The listing builds one solid part. Answer for the finished solid, in the listing's coordinates (mm). A direction names the side the tool comes from. Round coordinates to 2 decimals unless told otherwise and drop trailing zeros. Order: outer loops, then holes, each group sorted by start corner. A loop starts at its lowest first (then second) coordinate and runs counter-clockwise, first axis right, second up. Notation, with made-up numbers: M 83,36.5 L 127,36.5 A16 cw 127,56.5 Z; hole C -37.5,20 d4. An arc over 180 degrees is marked long. Put each result on its own line as item: value. Start each with the question number.
1. The part is cut by section D-D (x = 110). Give the vertices of the cut face in (y, z), then the cut area to 3 significant figures.
2. The part is cut by section C-C (z = 5). Give the vertices of the cut face in (x, y), then the cut area to 3 significant figures.
3. The part is cut by section B-B (x = 70). Give the vertices of the cut face in (y, z).
4. The part is cut by section A-A (x = 0). Give the vertices of the cut face in (y, z).
5. Consider line 1 (Y direction, x = 0, z = 11.55); line 2 (Z direction, x = 113, y = 2); line 3 (X direction, y = 1, z = -7.5). Determine where each line is inside the solid, lowest interval first.
6. Each of these flat-tipped pins is pushed along its axis until it touches: pin 1 Ø7 at (y, z) = (-3.5, -16) entering from +X; pin 2 Ø1.3 at (y, z) = (17, -11) entering from -X; pin 3 Ø1.5 at (y, z) = (5, -10) entering from -X. Where does it stop, or does it pass through?
7. Which of the six approach directions +Z, -Z, +X, -X, +Y, -Y give full straight-line access (tool end or side, diameter ignored) to faces 1 (the face through (-2, 5, -12.128)), 2 (the face through (-140.062, -2, -19)), 3 (the face through (140.062, -0.9, -18.2))?
8. The mould has two halves that part along Z. Classify faces 4 (the face through (-14.11, 16.78, 11.31)), 5 (the face through (-131, -6, -18.606)), 6 (the face through (-1, 6, 10.478)): +Z half, -Z half, draft (parallel to the pull), parting line (faces both ways), or undercut.
from build123d import *

# Parameters (mm, degrees)
BOSS_EXTRUDE1_DEPTH = 1.651
SKETCH2_W           = 18.415
SKETCH2_H           = 1.651
BOSS_EXTRUDE2_DEPTH = 10.287
FILLET1_R           = 2.54
FILLET3_R           = 1.27
SKETCH4_W           = 235.6739
SKETCH4_H           = 1.651
SKETCH4_W_2         = 286.8803
BOSS_EXTRUDE3_DEPTH = 30.861
SKETCH5_R           = 4.0005
CUT_EXTRUDE2_DEPTH  = 2.54
FILLET4_R           = 2.54
SKETCH11_R          = 5.207
CUT_EXTRUDE3_DEPTH  = 7.62


with BuildPart() as part:
    # Sketch1 → Boss-Extrude1 (new body)
    with BuildSketch(Plane(origin=(0, 0, 0), x_dir=(1, 0, 0), z_dir=(0, 1, 0))):
        with BuildLine():
            Line((117.83695, 8.5725), (117.83695, 12.1285))
            Line((117.83695, 12.1285), (117.186124302, 12.1285))
            Line((117.186124302, 12.1285), (-117.186124302, 12.1285))
            Line((-117.186124302, 12.1285), (-117.83695, 12.1285))
            Line((-117.83695, 12.1285), (-117.83695, 8.5725))
            ThreePointArc((-117.83695, 8.5725), (-119.74195, 6.6675), (-121.64695, 8.5725))
            Line((-121.64695, 8.5725), (-121.64695, 12.1285))
            Line((-121.64695, 12.1285), (-121.64695, 20.2565))
            Line((-121.64695, 20.2565), (-140.06195, 20.2565))
            Line((-140.06195, 20.2565), (-140.06195, 12.1285))
            Line((-140.06195, 12.1285), (-140.06195, 11.7475))
            ThreePointArc((-140.06195, 11.7475), (-140.433924388, 10.849474388), (-141.33195, 10.4775))
            Line((-141.33195, 10.4775), (-143.44015, 10.4775))
            Line((-143.44015, 10.4775), (-155.37815, 10.4775))
            Line((-155.37815, 10.4775), (-155.37815, -10.4775))
            Line((-155.37815, -10.4775), (-144.20215, -10.4775))
            ThreePointArc((-144.20215, -10.4775), (-143.663334633, -10.700684633), (-143.44015, -11.2395))
            Line((-143.44015, -11.2395), (-143.44015, -12.1285))
            Line((-143.44015, -12.1285), (143.44015, -12.1285))
            Line((143.44015, -12.1285), (143.44015, -11.2395))
            ThreePointArc((143.44015, -11.2395), (143.663334633, -10.700684633), (144.20215, -10.4775))
            Line((144.20215, -10.4775), (155.37815, -10.4775))
            Line((155.37815, -10.4775), (155.37815, 10.4775))
            Line((155.37815, 10.4775), (143.44015, 10.4775))
            Line((143.44015, 10.4775), (141.33195, 10.4775))
            ThreePointArc((141.33195, 10.4775), (140.433924388, 10.849474388), (140.06195, 11.7475))
            Line((140.06195, 11.7475), (140.06195, 12.1285))
            Line((140.06195, 12.1285), (140.06195, 20.2565))
            Line((140.06195, 20.2565), (121.64695, 20.2565))
            Line((121.64695, 20.2565), (121.64695, 12.1285))
            Line((121.64695, 12.1285), (121.64695, 8.5725))
            ThreePointArc((121.64695, 8.5725), (119.74195, 6.6675), (117.83695, 8.5725))
        make_face()
    extrude(amount=BOSS_EXTRUDE1_DEPTH)

    # Sketch2 → Boss-Extrude2 (add)
    with BuildSketch(Plane.XZ):
        with Locations((-130.85445, -19.431)):
            Rectangle(SKETCH2_W, SKETCH2_H)
        with Locations((130.85445, -19.431)):
            Rectangle(SKETCH2_W, SKETCH2_H)
    extrude(amount=BOSS_EXTRUDE2_DEPTH)

    # Fillet1
    fillet1_edges = [part.edges().sort_by_distance(p)[0] for p in [
        (130.85445, 1.651, -20.2565),
        (-130.85445, 1.651, -20.2565),
        (-130.85445, 0, -18.6055),
        (130.85445, 0, -18.6055),
    ]]
    fillet(fillet1_edges, radius=FILLET1_R)

    # Fillet3
    fillet3_edges = [part.edges().sort_by_distance(p)[0] for p in [
        (-140.06195, -10.287, -19.431),
        (-121.64695, -10.287, -19.431),
        (140.06195, -10.287, -19.431),
        (121.64695, -10.287, -19.431),
    ]]
    fillet(fillet3_edges, radius=FILLET3_R)

    # Sketch4 → Boss-Extrude3 (add)
    with BuildSketch(Plane(origin=(0, 1.651, 0), x_dir=(1, 0, 0), z_dir=(0, 1, 0))):
        with Locations((0, 11.303)):
            Rectangle(SKETCH4_W, SKETCH4_H)
        with Locations((0, -11.303)):
            Rectangle(SKETCH4_W_2, SKETCH4_H)
    extrude(amount=BOSS_EXTRUDE3_DEPTH)

    # Sketch5 → Cut-Extrude2 (cut)
    with BuildSketch(Plane.XY.offset(12.1285)):
        with Locations((0, 19.431)):
            Circle(SKETCH5_R)
        with BuildLine():
            Line((143.44015, 8.4582), (22.43455, 8.4582))
            Line((22.43455, 8.4582), (6.735192091, 24.157557909))
            ThreePointArc((6.735192091, 24.157557909), (0, 26.947365818), (-6.735192091, 24.157557909))
            Line((-6.735192091, 24.157557909), (-22.43455, 8.4582))
            Line((-22.43455, 8.4582), (-143.44015, 8.4582))
            Line((-143.44015, 8.4582), (-143.44015, 32.512))
            Line((-143.44015, 32.512), (143.44015, 32.512))
            Line((143.44015, 32.512), (143.44015, 8.4582))
        make_face()
    extrude(amount=-CUT_EXTRUDE2_DEPTH, mode=Mode.SUBTRACT)

    # Fillet4
    fillet4_edges = [part.edges().sort_by_distance(p)[0] for p in [
        (143.44015, 8.4582, 11.303),
        (22.43455, 8.4582, 11.303),
        (-22.43455, 8.4582, 11.303),
        (-143.44015, 8.4582, 11.303),
    ]]
    fillet(fillet4_edges, radius=FILLET4_R)

    # Sketch11 → Cut-Extrude3 (cut)
    with BuildSketch(Plane(origin=(0, 0, -12.1285), x_dir=(-1, 0, 0), z_dir=(0, 0, -1))):
        with Locations((60.68695, 19.812)):
            Circle(SKETCH11_R)
        with Locations((-60.68695, 19.812)):
            Circle(SKETCH11_R)
        with BuildLine():
            Line((81.00695, 8.4582), (117.83695, 8.4582))
            Line((117.83695, 8.4582), (117.83695, 32.512))
            Line((117.83695, 32.512), (60.68695, 32.512))
            ThreePointArc((60.68695, 32.512), (69.667206121, 28.792256121), (73.38695, 19.812))
            Line((73.38695, 19.812), (73.38695, 16.0782))
            ThreePointArc((73.38695, 16.0782), (75.618796327, 10.690046327), (81.00695, 8.4582))
        make_face()
        with BuildLine():
            Line((-28.742381637, 8.4582), (0, 8.4582))
            Line((0, 8.4582), (28.742381637, 8.4582))
            ThreePointArc((28.742381637, 8.4582), (31.172421432, 8.941564969), (33.232509697, 10.318071939))
            Line((33.232509697, 10.318071939), (51.706693879, 28.792256121))
            ThreePointArc((51.706693879, 28.792256121), (55.826870409, 31.545270063), (60.68695, 32.512))
            Line((60.68695, 32.512), (-60.68695, 32.512))
            ThreePointArc((-60.68695, 32.512), (-55.826870409, 31.545270063), (-51.706693879, 28.792256121))
            Line((-51.706693879, 28.792256121), (-33.232509697, 10.318071939))
            ThreePointArc((-33.232509697, 10.318071939), (-31.172421432, 8.941564969), (-28.742381637, 8.4582))
        make_face()
        with BuildLine():
            Line((-117.83695, 32.512), (-117.83695, 8.4582))
            Line((-117.83695, 8.4582), (-81.00695, 8.4582))
            ThreePointArc((-81.00695, 8.4582), (-75.618796327, 10.690046327), (-73.38695, 16.0782))
            Line((-73.38695, 16.0782), (-73.38695, 19.812))
            ThreePointArc((-73.38695, 19.812), (-69.667206121, 28.792256121), (-60.68695, 32.512))
            Line((-60.68695, 32.512), (-117.83695, 32.512))
        make_face()
    extrude(amount=-CUT_EXTRUDE3_DEPTH, mode=Mode.SUBTRACT)


solid = part.part
Resolved:
1. outline: M 0,-12.13 L 8.46,-12.13 L 8.46,-10.48 L 1.65,-10.48 L 1.65,10.48 L 8.46,10.48 L 8.46,12.13 L 0,12.13 Z
1. area: 62.5 mm2
2. outline: M -155.38,0 L 155.38,0 L 155.38,1.65 L -155.38,1.65 Z
2. area: 513 mm2
3. outline: M 0,-12.13 L 28.45,-12.13 L 28.45,-10.48 L 1.65,-10.48 L 1.65,10.48 L 8.46,10.48 L 8.46,12.13 L 0,12.13 Z
4. outline: M 0,-12.13 L 8.46,-12.13 L 8.46,-10.48 L 1.65,-10.48 L 1.65,10.48 L 15.43,10.48 L 15.43,12.13 L 0,12.13 Z; M 23.43,10.48 L 26.95,10.48 L 26.95,12.13 L 23.43,12.13 Z
5. line 1: 0 to 15.43, 23.43 to 26.95
5. line 2: -12.13 to -10.48, 10.48 to 12.13
5. line 3: -155.38 to -121.32, -118.17 to 118.17, 121.32 to 155.38
6. pin 1: x = 140.06
6. pin 2: x = -73.39
6. pin 3: x = -117.84
7. face 1: -Z, +Y, -Y
7. face 2: -Z, -X, +Y, -Y
7. face 3: -Z, +X, +Y, -Y
8. face 4: draft
8. face 5: +Z half
8. face 6: undercut
